Input: dimensioned drawing with shaded views. Units: mm. Origin: part minimum x, y, z. A direction names the side the tool comes from. Round coordinates to 2 decimals unless told otherwise and drop trailing zeros. Order: outer loops, then holes, each group sorted by start corner. A loop starts at its lowest first (then second) coordinate and runs counter-clockwise, first axis right, second up. Notation, with made-up numbers: M 32,59 L 81,59 A11 ccw 81,65 Z; hole C 51,15.25 d4. An arc over 180 degrees is marked long. Use one line per item in the form item = value. Start each with the question number.
Q1. Section D-D (z = 23.5). Return the cut outline in (x, y).
Q2. Reachability of the marked faces 4 and 5 from +Z, -Z, +X, -X, +Y, -Y: full face, straight path, thin tool, end or side. Return the list, or none.
Q3. Contact query for flat-ended pins moving along their axis: pin 1 (4 mm diameter, centred on x = 22, z = 55.5, fed in from +Y); pin 2 (23.5 mm diameter, centred on y = 42, z = 46, fed in from +X); pin 3 (6 mm diameter, centred on x = 21.5, y = 56.5, fed in from -Z); pin 4 (1.5 mm diameter, centred on y = 70, z = 60.5, fed in from +X). Output: stop coordinate, or through.
Q4. Material intervals for probe 1 along Y at (x, z) = (23, 39); probe 2 along Y at (x, z) = (7, 39); probe 3 along Z at (x, y) = (27, 65.5), sorted ascending.
Q5. Pull-direction query (Z, two-part tool) for the marked faces 1, 2 and 3; classes: pulls with the +Z half, pulls with the -Z half, needs draft (parallel to the pull), parting line crosses it, or undercut.
Q6. Section C-C (x = 32). Return the cut outline in (y, z).
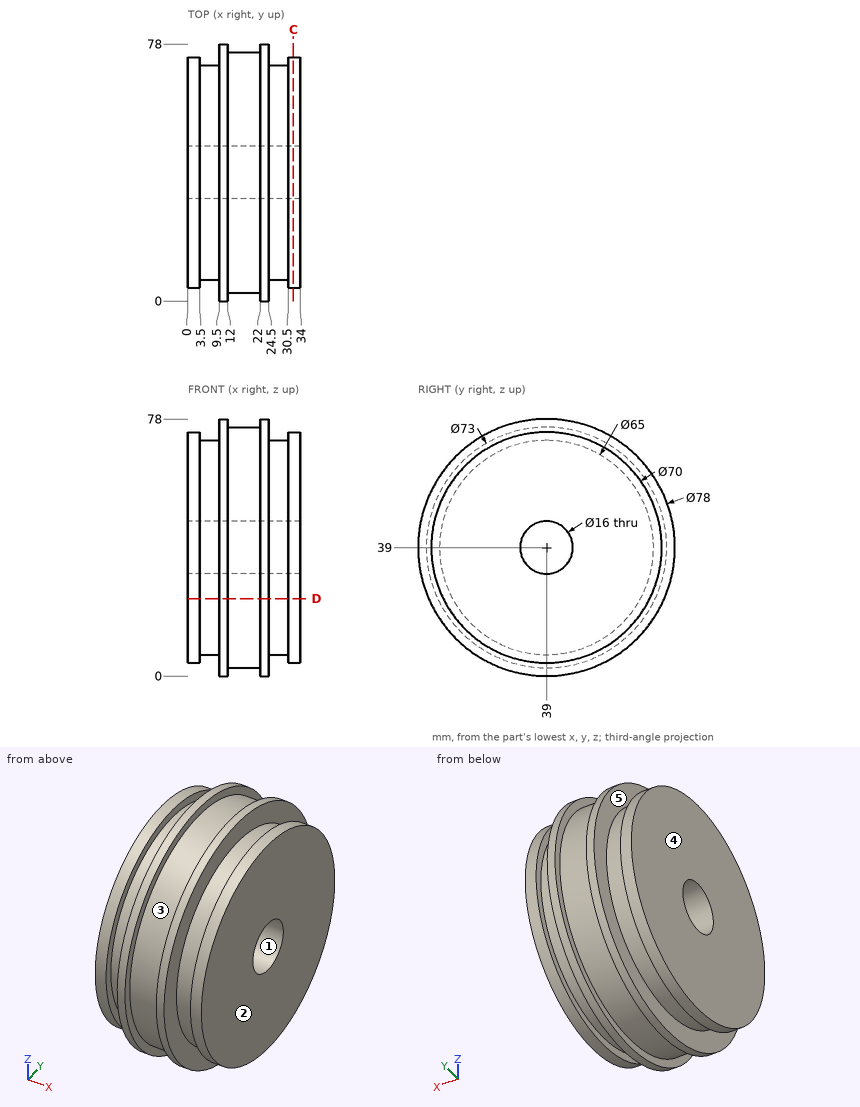
Results list:
q1.outline = M 0,7.62 L 3.5,7.62 L 3.5,10.43 L 9.5,10.43 L 9.5,3.21 L 12,3.21 L 12,5.95 L 22,5.95 L 22,3.21 L 24.5,3.21 L 24.5,10.43 L 30.5,10.43 L 30.5,7.62 L 34,7.62 L 34,70.38 L 30.5,70.38 L 30.5,67.57 L 24.5,67.57 L 24.5,74.79 L 22,74.79 L 22,72.05 L 12,72.05 L 12,74.79 L 9.5,74.79 L 9.5,67.57 L 3.5,67.57 L 3.5,70.38 L 0,70.38 Z
q2.face_4 = +Z, -Z, -X, +Y, -Y
q2.face_5 = none
q3.pin_1 = 75.2
q3.pin_2 = 34
q3.pin_3 = 2.81
q3.pin_4 = 24.5
q4.probe_1 = 0 to 31, 47 to 78
q4.probe_2 = 6.5 to 31, 47 to 71.5
q4.probe_3 = 20.19 to 57.81
q5.face_1 = undercut
q5.face_2 = needs draft
q5.face_3 = parting line crosses it
q6.outline = C 39,39 d70; hole C 39,39 d16
